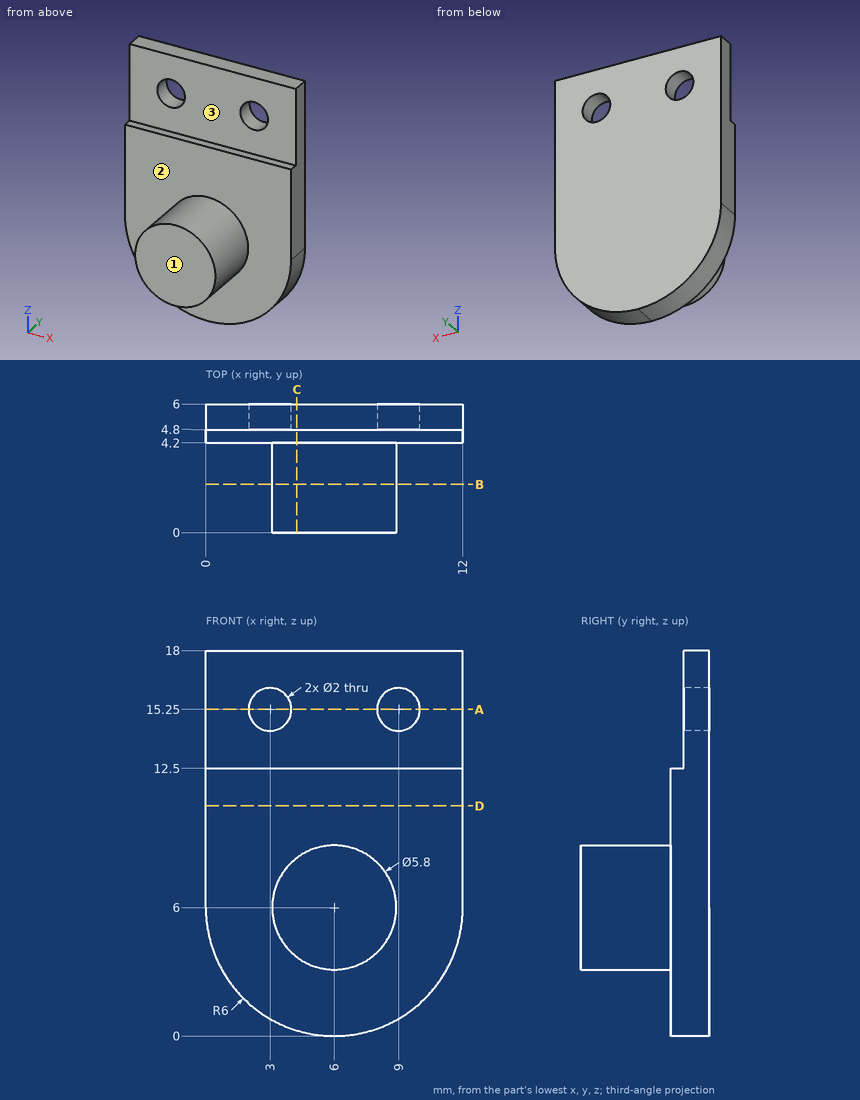
Input: dimensioned drawing with shaded views. Units: mm. Origin: part minimum x, y, z. A direction names the side the tool comes from. Give positions to 0.01 mm unless a question says otherwise; leave off trailing zeros. Write each loop counter-clockwise with the first axis right and the second up, starting at its lowest first coordinate (ties: lowest second). Pieces come first, ordered by that corner, then holes. Notation, with made-up numbers: (-10, 44) - (39, 44) arc R23 cw to (39, 72) - close; hole circle Ø11 at (6, -37). An arc over 180 degrees is marked (long way). Write item = value, one per line. Start each with the question number.
1) Material intervals for L1, parallel to Y at x = 10, z = 2; L2, parallel to X at y = 5.2, z = 14.75; L3, parallel to Y at x = 1, z = 15, sorted ascending. Write a range as [from, to].
2) Reachability of the marked faces 1, 2 and 3 from +Z, -Z, +X, -X, +Y, -Y: full face, straight path, thin tool, end or side. Return the list, or none.
3) Cut plane C-C (x = 4.25). Return loops of the section in (y, z).
4) Cut plane A-A (z = 15.25). Return loops of the section in (x, y), and give its area (3 significant figures).
5) Cut plane D-D (z = 10.75). Return loops of the section in (x, y), and give its area (3 significant figures).
6) Cut plane B-B (y = 2.25). Return loops of the section in (x, z).
7) Pin query (flat end, axial travel): pin 1 (1.5 mm diameter, centred on x = 8, y = 4, fed in from +Z); pin 2 (1 mm diameter, centred on y = 1, z = 3, fed in from +X); pin 3 (2.5 mm diameter, centred on x = 3, z = 15.25, fed in from -Y). Return the tip coordinate at first contact, or that it passes through.
Answers follow:
q1.L1 = [4.2, 6]
q1.L2 = [0, 2.13], [3.87, 8.13], [9.87, 12]
q1.L3 = [4.8, 6]
q2.face_1 = +Z, -Z, +X, -X, -Y
q2.face_2 = -Y
q2.face_3 = +Z, +X, -X, -Y
q3.outline = (0, 3.69) - (4.2, 3.69) - (4.2, 0.26) - (6, 0.26) - (6, 18) - (4.8, 18) - (4.8, 12.5) - (4.2, 12.5) - (4.2, 8.31) - (0, 8.31) - close
q4.outline = (0, 4.8) - (2, 4.8) - (2, 6) - (0, 6) - close; (4, 4.8) - (8, 4.8) - (8, 6) - (4, 6) - close; (10, 4.8) - (12, 4.8) - (12, 6) - (10, 6) - close
q4.area = 9.60 mm^2
q5.outline = (0, 4.2) - (12, 4.2) - (12, 6) - (0, 6) - close
q5.area = 21.6 mm^2
q6.outline = circle Ø5.8 at (6, 6)
q7.pin_1 = 12.5
q7.pin_2 = 7.47
q7.pin_3 = 4.8
